from build123d import *

# Parameters (mm, degrees)
SCHIZZO1_R                   = 22.5
SCHIZZO1_R_2                 = 9
ESTRUSIONE_ESTRUSIONE1_DEPTH = 30
SCHIZZO3_R                   = 3
ESTRUSIONE_ESTRUSIONE2_DEPTH = 25
SCHIZZO4_R                   = 9
TAGLIO_ESTRUSIONE1_DEPTH     = 40


with BuildPart() as part:
    # Schizzo1 → Estrusione-Estrusione1 (new body)
    with BuildSketch(Plane.XY):
        Circle(SCHIZZO1_R)
        Circle(SCHIZZO1_R_2, mode=Mode.SUBTRACT)
    extrude(amount=ESTRUSIONE_ESTRUSIONE1_DEPTH)

    # Schizzo3 → Estrusione-Estrusione2 (add)
    with BuildSketch(Plane(origin=(0, 0, 0), x_dir=(1, 0, 0), z_dir=(0, 1, 0))):
        with Locations((0, -10)):
            Circle(SCHIZZO3_R)
    extrude(amount=-ESTRUSIONE_ESTRUSIONE2_DEPTH)

    # Schizzo4 → Taglio-Estrusione1 (cut)
    with BuildSketch(Plane.XY.offset(30)):
        Circle(SCHIZZO4_R)
    extrude(amount=-TAGLIO_ESTRUSIONE1_DEPTH, mode=Mode.SUBTRACT)


solid = part.part
Work out the finished part from the listing and answer in its coordinate system (mm). A direction names the side the tool comes from. Give positions to 0.01 mm unless a question says otherwise; leave off trailing zeros. Write each loop counter-clockwise with the first axis right and the second up, starting at its lowest first coordinate (ties: lowest second). Pieces come first, ordered by that corner, then holes. Notation, with made-up numbers: (38, 42.5) - (42, 42.5) arc R13 cw to (42, 60.5) - close; hole circle Ø5 at (-5.75, 58.5). An arc over 180 degrees is marked (long way). One line per item, written item: value. Start each with the question number.
1. Find section D-D (x = -6). Write down the section's boundary in (y, z), then the cut area to 3 significant figures.
2. Given pin 1 (1 mm diameter, centred on x = 1, z = 20, fed in from +Y); pin 2 (4 mm diameter, centred on y = 15.5, z = 17, fed in from +X); pin 3 (2 mm diameter, centred on y = 8.5, z = 5, fed in from -X); pin 4 (4 mm diameter, centred on x = -9.5, y = -9.5, fed in from -Z), each flat-ended and moving along its own axis, determine where each tip first touches the part or whether it passes through.
3. Consider probe 1 along Y at (x, z) = (0, 12); probe 2 along Y at (x, z) = (0, 21.5); probe 3 along X at (y, z) = (-4.5, 7). Determine where each line is inside the solid, lowest interval first.
4. Find section B-B (y = 0). Write down the section's boundary in (x, z), then the cut area to 3 significant figures.
5. Find section A-A (x = 0). Write down the section's boundary in (y, z).
6. For faces 1 (the cylindrical face through (-3, -24, 10)), 2 (the flat face through (10, 0, 30)), determine the directions among +Z, -Z, +X, -X, +Y, -Y from which every point of the face is accessible in a straight line to the end or side of a thin tool.
7. Find section C-C (z = 10). Write down the section's boundary in (x, y).
Geometry results:
1. outline: (-21.69, 0) - (-6.71, 0) - (-6.71, 30) - (-21.69, 30) - close; (6.71, 0) - (21.69, 0) - (21.69, 30) - (6.71, 30) - close
1. area: 899 mm2
2. pin 1: y = 22.49
2. pin 2: x = 18
2. pin 3: x = -21.21
2. pin 4: z = 0
3. probe 1: -25 to -9, 9 to 22.5
3. probe 2: -22.5 to -9, 9 to 22.5
3. probe 3: -22.05 to -7.79, 7.79 to 22.05
4. outline: (-22.5, 0) - (-9, 0) - (-9, 30) - (-22.5, 30) - close; (9, 0) - (22.5, 0) - (22.5, 30) - (9, 30) - close
4. area: 810 mm2
5. outline: (-25, 7) - (-22.5, 7) - (-22.5, 0) - (-9, 0) - (-9, 30) - (-22.5, 30) - (-22.5, 13) - (-25, 13) - close; (9, 0) - (22.5, 0) - (22.5, 30) - (9, 30) - close
6. face 1: -Y
6. face 2: +Z, +X, -X, +Y, -Y
7. outline: (-3, -25) - (3, -25) - (3, -22.3) arc R22.5 ccw (long way) to (-3, -22.3) - close; hole circle Ø18 at (0, 0)
